Input: part model. Units: mm. Frame: model coordinates. Round coordinates to 2 decimals unless told otherwise and drop trailing zeros. Loops run counter-clockwise (first coordinate to the right, second up) from the corner with the lowest first, then second, coordinate; pieces in that order, holes last. Notation, with made-up numbers: M -14.75,14 L 12.25,14 A22 cw 12.25,47 Z; hole C -35,3 d6. An arc over 180 degrees is marked long. Put each result on its own line as item: value. Start each with the question number.
1) Section C-C on x = 139. Output: boundary loops of the cut face in (y, z).
2) Line query: probe 1 along Y at (x, z) = (137, 45.5); probe 2 along Y at (x, z) = (151.5, 43.25); probe 3 along Y at (x, z) = (155.5, 41.5). Output: solid intervals per line, ascending.
3) Pin query (flat end, axial travel): pin 1 (4.5 mm diameter, centred on x = 153.59, y = 275.68, fed in from +Z) (3 decimals). Return the tip coordinate at first contact, or that it passes through.
4) Section A-A on x = 122.5. Output: boundary loops of the cut face in (y, z).
5) Section B-B on y = 283. Output: boundary loops of the cut face in (x, z).
6) Draft query along Y for faces 1 (the face through (127.87, 300.62, 43.46)), 2 (the face through (137, 314.676, 43)), 3 (the face through (153.247, 311.254, 43.458)), 4 (the face through (147, 282, 36.731)). Return one class per face: +Y half, -Y half, draft (parallel to the pull), parting line (faces both ways), or undercut.
7) Section D-D on y = 308. Output: boundary loops of the cut face in (x, z), plus the area to 3 significant figures.
from build123d import *

# Parameters (mm, degrees)
EXTRUDE_1_DEPTH     = 13.268852707
SKETCH_2_R          = 2.6
CUT_EXTRUDE_1_DEPTH = 30
SKETCH_3_R          = 12.5
CUT_EXTRUDE_2_DEPTH = 30


with BuildPart() as part:
    # Эскиз1 → Бобышка-Вытянуть1 (new body)
    with BuildSketch(Plane.XY.offset(36.731147293)):
        with BuildLine():
            Line((114.085323537, 309.675869107), (114.085323537, 274.675869107))
            ThreePointArc((114.085323537, 274.675869107), (115.549789632, 271.140335201), (119.085323537, 269.675869107))
            Line((119.085323537, 269.675869107), (155.085323537, 269.675869107))
            ThreePointArc((155.085323537, 269.675869107), (158.620857443, 271.140335201), (160.085323537, 274.675869107))
            Line((160.085323537, 274.675869107), (160.085323537, 309.675869107))
            ThreePointArc((160.085323537, 309.675869107), (158.620857443, 313.211403013), (155.085323537, 314.675869107))
            Line((155.085323537, 314.675869107), (119.085323537, 314.675869107))
            ThreePointArc((119.085323537, 314.675869107), (115.549789632, 313.211403013), (114.085323537, 309.675869107))
        make_face()
    extrude(amount=EXTRUDE_1_DEPTH)

    # Эскиз2 → Вырез-Вытянуть1 (cut)
    with BuildSketch(Plane.XY.offset(50)):
        with Locations((153.585323537, 308.675869107)):
            Circle(SKETCH_2_R)
        with Locations((120.585323537, 308.675869107)):
            Circle(SKETCH_2_R)
        with Locations((120.585323537, 275.675869107)):
            Circle(SKETCH_2_R)
        with Locations((153.585323537, 275.675869107)):
            Circle(SKETCH_2_R)
    extrude(amount=-CUT_EXTRUDE_1_DEPTH, mode=Mode.SUBTRACT)

    # Эскиз3 → Вырез-Вытянуть2 (cut)
    with BuildSketch(Plane.XY.offset(50)):
        with Locations((137.085323537, 292.175869107)):
            Circle(SKETCH_3_R)
    extrude(amount=-CUT_EXTRUDE_2_DEPTH, mode=Mode.SUBTRACT)


solid = part.part
Geometry results:
1. outline: M 269.68,36.73 L 279.82,36.73 L 279.82,50 L 269.68,50 Z; M 304.53,36.73 L 314.68,36.73 L 314.68,50 L 304.53,50 Z
2. probe 1: y = 269.68 to 279.68, 304.68 to 314.68
2. probe 2: y = 269.68 to 274.12, 277.23 to 307.12, 310.23 to 314.68
2. probe 3: y = 269.69 to 273.92, 277.43 to 306.92, 310.43 to 314.66
3. pin 1: passes through
4. outline: M 269.68,36.73 L 273.92,36.73 L 273.92,50 L 269.68,50 Z; M 277.43,36.73 L 306.92,36.73 L 306.92,50 L 277.43,50 Z; M 310.43,36.73 L 314.68,36.73 L 314.68,50 L 310.43,50 Z
5. outline: M 114.09,36.73 L 128.6,36.73 L 128.6,50 L 114.09,50 Z; M 145.57,36.73 L 160.09,36.73 L 160.09,50 L 145.57,50 Z
6. face 1: undercut
6. face 2: +Y half
6. face 3: undercut
6. face 4: draft
7. outline: M 114.09,36.73 L 118.07,36.73 L 118.07,50 L 114.09,50 Z; M 123.1,36.73 L 151.07,36.73 L 151.07,50 L 123.1,50 Z; M 156.1,36.73 L 160.09,36.73 L 160.09,50 L 156.1,50 Z
7. area: 477 mm²
